The listing builds one solid part. Answer for the finished solid, in the listing's coordinates (mm). Face numbers are marked on the shaded views. A direction names the side the tool comes from. Coordinates: 2 decimals unless noted, no trailing zeros. Order: outer loops, then holes, each group sorted by start corner. A loop starts at its lowest first (then second) coordinate and runs counter-clockwise, first axis right, second up. Notation, with made-up numbers: (56.25, 19.25) -> (89.25, 19.25) arc R26 ccw to (89.25, 49.25) -> close; hole circle Ø6 at (-6, -1.5). An arc over 180 degrees is marked (long way). Answer in a Markdown table with one row per item. Add a question column.
```python
from build123d import *

# Parameters (mm, degrees)
SKIZZE1_W                       = 4
SKIZZE1_H                       = 20
SKIZZE5_W                       = 10
SKIZZE5_H                       = 10
AUFSATZ_LINEAR_AUSTRAGEN1_DEPTH = 10
SKETCH1_R                       = 2.5
CUT_EXTRUDE1_DEPTH              = 31.822070015


with BuildPart() as part:
    # Skizze1 → Rotation1 (revolve)
    with BuildSketch(Plane.XY, mode=Mode.PRIVATE) as rotation1_sk:
        with Locations((2, 10)):
            Rectangle(SKIZZE1_W, SKIZZE1_H)
    revolve(rotation1_sk.sketch.rotate(Axis((0, -2.459302686, 0), (0, 1, 0)), 90), axis=Axis((0, -2.459302686, 0), (0, 1, 0)))

    # Skizze5 → Aufsatz-Linear austragen1 (add)
    with BuildSketch(Plane(origin=(0, 20, 0), x_dir=(1, 0, 0), z_dir=(0, 1, 0))):
        Rectangle(SKIZZE5_W, SKIZZE5_H)
    extrude(amount=AUFSATZ_LINEAR_AUSTRAGEN1_DEPTH)

    # Sketch1 → Cut-Extrude1 (cut, through all)
    with BuildSketch(Plane(origin=(0, 30, 0), x_dir=(1, 0, 0), z_dir=(0, 1, 0))):
        with Locations(Location((0, 0, 0), (0, 0, 270))):
            Circle(SKETCH1_R)
    extrude(amount=-CUT_EXTRUDE1_DEPTH, mode=Mode.SUBTRACT)


solid = part.part
```
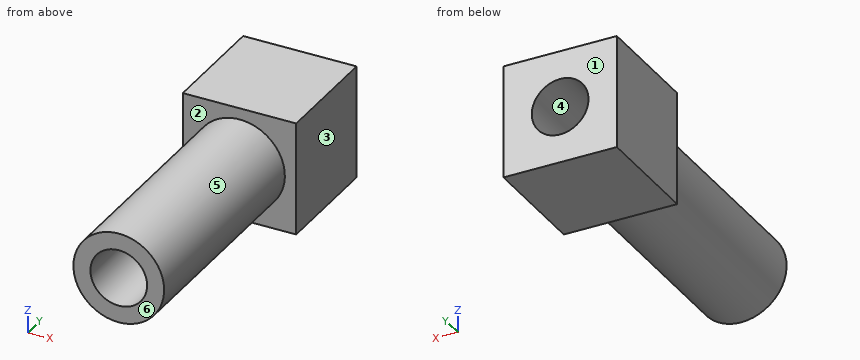
Q1. Determine the mould class of the marked faces 3, 4, 5 and 6 for opening direction X: +X half, -X half, draft (parallel to the pull), parting line (faces both ways), or undercut.
Q2. A cutting plane is placed at B-B (x = 0). Determine the outline of the cut face in (y, z).
Q3. A cutting plane is placed at D-D (x = -3). Determine the outline of the cut face in (y, z).
Q4. Given pin 1 (3 mm diameter, centred on x = -3.5, y = 10.5, fed in from +Z); pin 2 (5 mm diameter, centred on x = -0.5, y = 6.5, fed in from -Z), each flat-ended and moving along its own axis, determine where each tip first touches the part or whether it passes through.
Q5. A cutting plane is placed at A-A (z = 0). Determine the outline of the cut face in (x, y).
Q6. Straight lines are drawn through the part: line 1 (X direction, y = 19.5, z = 0); line 2 (X direction, y = 22.5, z = 0); line 3 (Y direction, x = -4, z = 1). For each, find the intervals that lie inside material, in ascending order.
Q7. A cutting plane is placed at C-C (y = 26.75). Determine the outline of the cut face in (x, z).
Q8. For the marked faces 1 and 2, determine the directions among +Z, -Z, +X, -X, +Y, -Y from which every point of the face is accessible in a straight line to the end or side of a thin tool.
Returned:
| question | item | result |
|---|---|---|
| 1 | face 3 | +X half |
| 1 | face 4 | undercut |
| 1 | face 5 | parting line |
| 1 | face 6 | draft |
| 2 | outline | (0, -4) -> (20, -4) -> (20, -5) -> (30, -5) -> (30, -2.5) -> (0, -2.5) -> close; (0, 2.5) -> (30, 2.5) -> (30, 5) -> (20, 5) -> (20, 4) -> (0, 4) -> close |
| 3 | outline | (0, -2.65) -> (20, -2.65) -> (20, -5) -> (30, -5) -> (30, 5) -> (20, 5) -> (20, 2.65) -> (0, 2.65) -> close |
| 4 | pin 1 | stops at z = 3.46 |
| 4 | pin 2 | stops at z = -4 |
| 5 | outline | (-5, 20) -> (-4, 20) -> (-4, 0) -> (-2.5, 0) -> (-2.5, 30) -> (-5, 30) -> close; (2.5, 0) -> (4, 0) -> (4, 20) -> (5, 20) -> (5, 30) -> (2.5, 30) -> close |
| 6 | line 1 | x = -4 to -2.5, 2.5 to 4 |
| 6 | line 2 | x = -5 to -2.5, 2.5 to 5 |
| 6 | line 3 | y = 20 to 30 |
| 7 | outline | (-5, -5) -> (5, -5) -> (5, 5) -> (-5, 5) -> close; hole circle Ø5 at (0, 0) |
| 8 | face 1 | +Z, -Z, +X, -X, +Y |
| 8 | face 2 | -Y |
